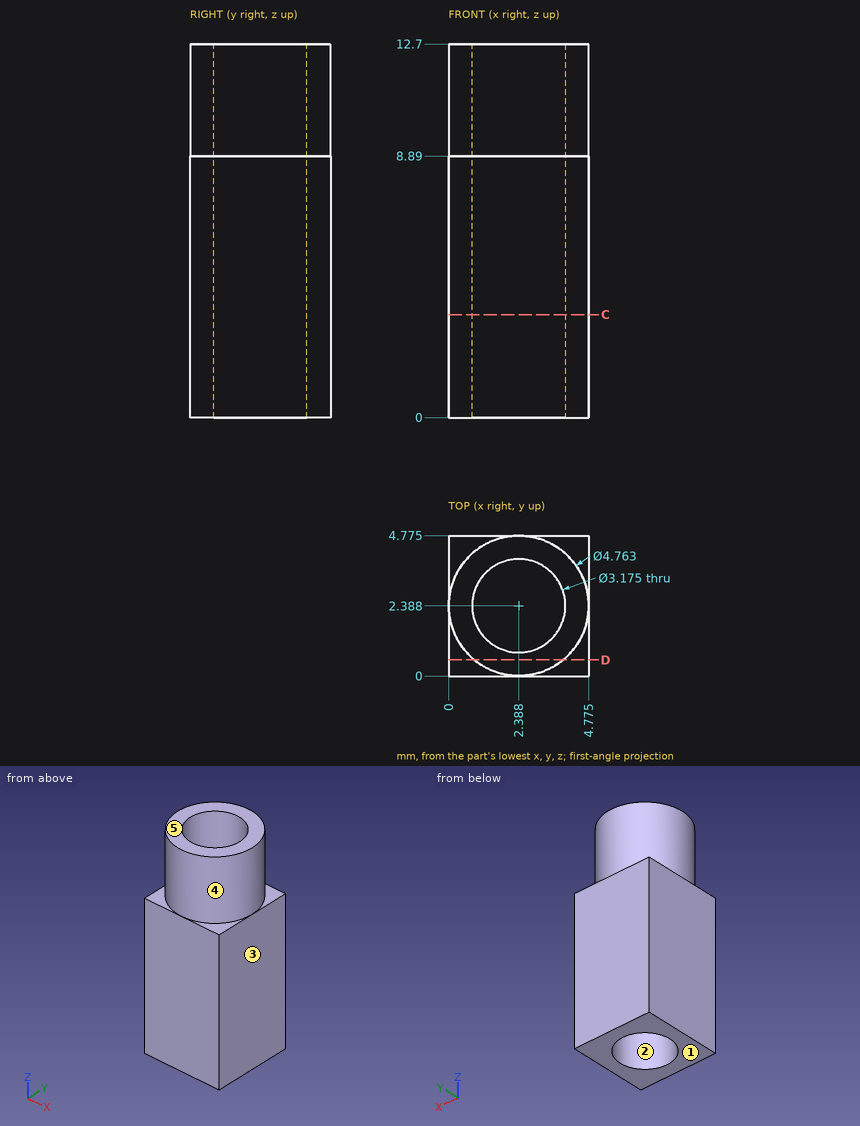
Geometry: see drawing. Coordinates: mm, zero at the bounding-box minimum. A direction names the side the tool comes from. Give positions to 0.01 mm unless a question says otherwise; leave off trailing zeros. Write each loop counter-clockwise with the first axis right and the second up, starting at its lowest first coordinate (ties: lowest second). Pieces come first, ordered by that corner, then holes. Notation, with made-up numbers: M -4,-0.5 L 12,-0.5 A32 ccw 12,34.5 Z; hole C 17,4 d6. An arc over 180 degrees is marked long. Return JSON: item names as keys, results as strings. Group by question number.
1) Ray query, L1, parallel to Z at x = 4.2, y = 4.45; L2, parallel to X at y = 0.95, z = 2 (1 decimal); L3, parallel to Y at x = 1.6, z = 3.25 (1 decimal). Return the intervals inside material, ascending.
2) First-contact query: pin 1 Ø1 at (x, z) = (4, 6.5) entering from -Y; pin 2 Ø1 at (x, y) = (2.5, 3) entering from +Z. Flat tips, straight axial feed; report the tip coordinate or a pass-through.
3) Cut plane D-D, the plane y = 0.55. Output: boundary loops of the cut face in (x, z) (1 decimal), then the cut area to 3 significant figures.
4) Draft query along X for the marked faces 1, 2 and 3. Return one class per face: released by +X, released by -X, zero draft, split by the parting line, or undercut.
5) Set-up query: the marked faces 4 and 5. Return all of +Z, -Z, +X, -X, +Y, -Y with unobstructed straight access to the full face (end or side cutting, diameter ignored); none if empty.
6) Cut plane C-C, the plane z = 3.5. Output: boundary loops of the cut face in (x, y) (1 decimal).
Data:
{
 "1": {"L1": "z = 0 to 8.89", "L2": "x = 0 to 1.7, 3.1 to 4.8", "L3": "y = 0 to 1, 3.8 to 4.8"},
 "2": {"pin 1": "stops at y = 0", "pin 2": "passes through"},
 "3": {"outline": "M 0,0 L 4.8,0 L 4.8,8.9 L 3.9,8.9 L 3.9,12.7 L 0.9,12.7 L 0.9,8.9 L 0,8.9 Z", "area": "54.0 mm²"},
 "4": {"face 1": "zero draft", "face 2": "undercut", "face 3": "released by +X"},
 "5": {"face 4": "+Z", "face 5": "+Z, +X, -X, +Y, -Y"},
 "6": {"outline": "M 0,0 L 4.8,0 L 4.8,4.8 L 0,4.8 Z; hole C 2.4,2.4 d3.2"}
}
